Geometry: see drawing. Coordinates: mm, zero at the bounding-box minimum. Give positions to 0.01 mm unless a question says otherwise; leave off trailing zeros. Write each loop counter-clockwise with the first axis right and the second up, starting at its lowest first coordinate (ties: lowest second). Pieces come first, ordered by that corner, then holes. Notation, with made-up numbers: (63, 80) - (80, 80) arc R31 ccw to (80, 108) - close; hole circle Ø6 at (26, 72). An arc over 180 degrees is marked (long way). Return JSON: item names as keys, results as strings.
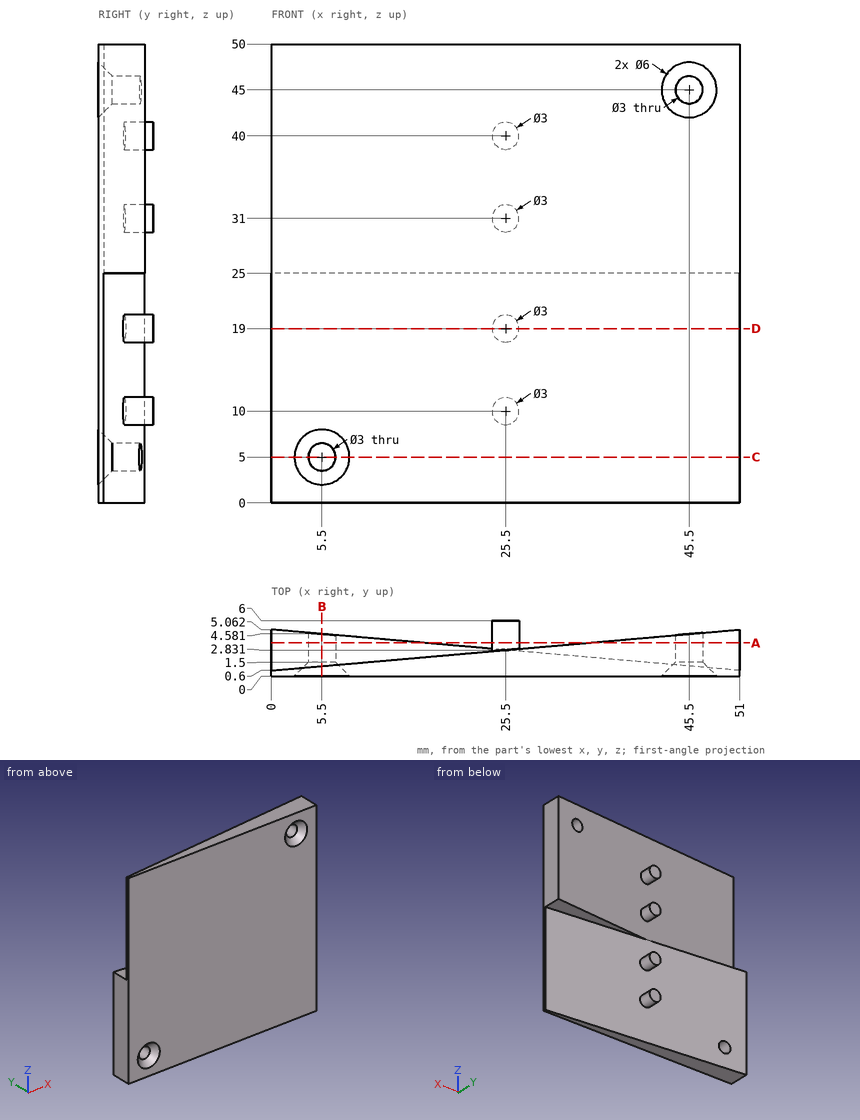
Q1. Section query B-B, the plane x = 5.5. Return the cut outline in (y, z).
Answer key:
{"outline": "(0, 0) - (4.58, 0) - (4.58, 3.5) - (1.5, 3.5) - (0, 2) - close; (0, 8) - (1.5, 6.5) - (4.58, 6.5) - (4.58, 25) - (1.08, 25) - (1.08, 50) - (0, 50) - close"}
Q2. Section query D-D, the plane z = 19. Return the cut outline in (x, y), plus the area to 3 significant figures.
Answer key:
{"outline": "(0, 0) - (51, 0) - (51, 0.6) - (27, 2.7) - (27, 6) - (24, 6) - (24, 2.96) - (0, 5.06) - close", "area": "154 mm^2"}
Q3. Section query A-A, the plane y = 3.6. Return the cut outline in (x, z).
Answer key:
{"outline": "(0, 0) - (16.71, 0) - (16.71, 25) - (0, 25) - close; circle Ø3 at (25.5, 10); circle Ø3 at (25.5, 19); circle Ø3 at (25.5, 31); circle Ø3 at (25.5, 40); (34.29, 25) - (51, 25) - (51, 50) - (34.29, 50) - close; hole circle Ø3 at (5.5, 5); hole circle Ø3 at (45.5, 45)"}
Q4. Pin query (flat end, axial travel): P1, Ø1.3, axis at x = 10, y = 3, coming from the +Z side; P2, Ø4, axis at x = 5.5, z = 5, coming from the -Y side. Return the tip coordinate at first contact, or that it passes through.
Answer key:
{"P1": "stops at z = 25", "P2": "stops at y = 1"}
Q5. Material intervals for probe 1 along Z at (x, y) = (45.5, 3.55); probe 2 along Z at (x, y) = (48.5, 2.6); probe 3 along X at (y, z) = (0.5, 6), sorted ascending. Write a range as [from, to].
Answer key:
{"probe 1": "z = [25, 43.5], [46.5, 50]", "probe 2": "z = [25, 50]", "probe 3": "x = [0, 3.21], [7.79, 51]"}
Q6. Section query C-C, the plane z = 5. Return the cut outline in (x, y).
Answer key:
{"outline": "(0, 0) - (2.5, 0) - (4, 1.5) - (4, 4.71) - (0, 5.06) - close; (7, 1.5) - (8.5, 0) - (51, 0) - (51, 0.6) - (7, 4.45) - close"}
